```python
from build123d import *
from build123d.topology import SkipClean

# Parameters (mm, degrees)
SKETCH1_W           = 10
SKETCH1_H           = 16
BOSS_EXTRUDE1_DEPTH = 8
FILLET1_R           = 4
SKETCH2_R           = 1.5
CUT_EXTRUDE1_DEPTH  = 16
SKETCH3_W           = 51
SKETCH3_H           = 16
BOSS_EXTRUDE2_DEPTH = 8
SKETCH4_W           = 36
SKETCH4_H           = 16
BOSS_EXTRUDE3_DEPTH = 4.5
SKETCH6_R           = 10.5
CUT_EXTRUDE6_DEPTH  = 16
SKETCH11_W          = 3
SKETCH11_H          = 16
BOSS_EXTRUDE4_DEPTH = 4.5
FILLET3_R           = 4
BOSS_EXTRUDE5_DEPTH = 1
SKETCH14_R          = 1.75
CUT_EXTRUDE7_DEPTH  = 1
BOSS_EXTRUDE6_DEPTH = 5
FILLET4_R           = 6.5
FILLET5_R           = 0.5
FILLET6_R           = 4
FILLET7_R           = 0.5
SKETCH17_W          = 51
SKETCH17_H          = 12.2
CUT_EXTRUDE9_DEPTH  = 6
SKETCH18_R          = 0.5
CUT_EXTRUDE10_DEPTH = 8


# Some blends are built 0.0001 mm under size
with BuildPart() as part:
    # Sketch1 → Boss-Extrude1 (new body)
    with BuildSketch(Plane(origin=(0, 0, 0), x_dir=(1, 0, 0), z_dir=(0, 1, 0))):
        Rectangle(SKETCH1_W, SKETCH1_H)
    extrude(amount=BOSS_EXTRUDE1_DEPTH)

    # Fillet1
    fillet1_edges = [part.edges().sort_by_distance(p)[0] for p in [
        (5, 0, 0),
        (5, 8, 0),
    ]]
    fillet(fillet1_edges, radius=FILLET1_R - 0.0001)  # a hair under: the kernel refuses the full size

    # Sketch2 → Cut-Extrude1 (cut)
    with BuildSketch(Plane.XY.offset(8)):
        with Locations((1, 4)):
            Circle(SKETCH2_R)
    extrude(amount=-CUT_EXTRUDE1_DEPTH, mode=Mode.SUBTRACT)

    # Sketch3 → Boss-Extrude2 (add)
    with BuildSketch(Plane(origin=(0, 0, 0), x_dir=(1, 0, 0), z_dir=(0, 1, 0))):
        with Locations((-30.5, 0)):
            Rectangle(SKETCH3_W, SKETCH3_H)
    extrude(amount=BOSS_EXTRUDE2_DEPTH)

    # Sketch4 → Boss-Extrude3 (add)
    with BuildSketch(Plane(origin=(0, 0, 0), x_dir=(1, 0, 0), z_dir=(0, 1, 0))):
        with Locations((-74, 0)):
            Rectangle(SKETCH4_W, SKETCH4_H)
    extrude(amount=BOSS_EXTRUDE3_DEPTH)

    # Sketch6 → Cut-Extrude6 (cut)
    with BuildSketch(Plane(origin=(0, 4.5, 0), x_dir=(1, 0, 0), z_dir=(0, 1, 0))):
        with Locations((-81.5, 0)):
            Circle(SKETCH6_R)
    extrude(amount=-CUT_EXTRUDE6_DEPTH, mode=Mode.SUBTRACT)


with BuildPart() as cut_extrude6_piece_1:
    # of the separate pieces the step leaves, piece 1, a body of its own (cut_extrude6_pieces)
    add(part.part.solids().sort_by_distance((5, 3.9999, -8))[0])



with BuildPart() as cut_extrude6_piece_2:
    # of the separate pieces the step leaves, piece 2, a body of its own (cut_extrude6_pieces)
    add(part.part.solids().sort_by_distance((-88.300735254, 4.5, 8))[0])



with BuildPart() as cut_extrude6_piece_3:
    # of the separate pieces the step leaves, piece 3, a body of its own (cut_extrude6_pieces)
    add(part.part.solids().sort_by_distance((-88.300735254, 0, -8))[0])


with BuildPart() as cut_extrude6_piece_2_1:
    add(cut_extrude6_piece_2.part)

    add(cut_extrude6_piece_3.part)  # Boss-Extrude4 merges Cut-Extrude6 piece 3
    # Sketch11 → Boss-Extrude4 (add)
    with BuildSketch(Plane(origin=(0, 0, 0), x_dir=(1, 0, 0), z_dir=(0, 1, 0))):
        with Locations((-93.5, 0)):
            Rectangle(SKETCH11_W, SKETCH11_H)
    extrude(amount=BOSS_EXTRUDE4_DEPTH)

    # Fillet3
    fillet3_edges = [cut_extrude6_piece_2_1.edges().sort_by_distance(p)[0] for p in [
        (-95, 2.25, 8),
        (-95, 2.25, -8),
    ]]
    fillet(fillet3_edges, radius=FILLET3_R)


with BuildPart() as cut_extrude6_piece_1_1:
    add(cut_extrude6_piece_1.part)

    add(cut_extrude6_piece_2_1.part)  # Boss-Extrude5 merges Cut-Extrude6 piece 2
    # Sketch13 → Boss-Extrude5 (add)
    with BuildSketch(Plane(origin=(0, 4.5, 0), x_dir=(1, 0, 0), z_dir=(0, 1, 0))):
        with BuildLine():
            Line((-88.300735254, 8), (-91, 8))
            ThreePointArc((-91, 8), (-93.828427125, 6.828427125), (-95, 4))
            Line((-95, 4), (-95, -4))
            ThreePointArc((-95, -4), (-93.828427125, -6.828427125), (-91, -8))
            Line((-91, -8), (-88.300735254, -8))
            Line((-88.300735254, -8), (-74.699264746, -8))
            Line((-74.699264746, -8), (-56, -8))
            Line((-56, -8), (-56, 8))
            Line((-56, 8), (-74.699264746, 8))
            Line((-74.699264746, 8), (-88.300735254, 8))
        make_face()
    extrude(amount=BOSS_EXTRUDE5_DEPTH)

    # Sketch14 → Cut-Extrude7 (cut)
    with BuildSketch(Plane(origin=(0, 5.5, 0), x_dir=(1, 0, 0), z_dir=(0, 1, 0))):
        with Locations(Location((-81.5, 0, 0), (0, 0, 270))):
            Circle(SKETCH14_R)
    extrude(amount=-CUT_EXTRUDE7_DEPTH, mode=Mode.SUBTRACT)

    # Sketch15 → Boss-Extrude6 (add)
    with SkipClean():  # the faces are left unmerged after this step: merging them gives an invalid solid
        with BuildSketch(Plane.XZ):
            with BuildLine():
                Line((-91, 8), (-88.300735254, 8))
                ThreePointArc((-88.300735254, 8), (-92, 0), (-88.300735254, -8))
                Line((-88.300735254, -8), (-91, -8))
                ThreePointArc((-91, -8), (-93.828427125, -6.828427125), (-95, -4))
                Line((-95, -4), (-95, 4))
                ThreePointArc((-95, 4), (-93.828427125, 6.828427125), (-91, 8))
            make_face()
            with BuildLine():
                Line((-71.895313644, 8), (-74.699264746, 8))
                ThreePointArc((-74.699264746, 8), (-71, 0), (-74.699264746, -8))
                Line((-74.699264746, -8), (-71.895313644, -8))
                ThreePointArc((-71.895313644, -8), (-69, 0), (-71.895313644, 8))
            make_face()
        extrude(amount=BOSS_EXTRUDE6_DEPTH)

    # Fillet4
    # the kernel refuses this fillet: 6.5 mm, written as the material it takes off along each edge
    with BuildSketch(Plane(origin=(-81.5, -5, 0), x_dir=(-0.06203986114443866, 0, -0.998073672445666), z_dir=(-0.998073672445666, 0, 0.06203986114443866))) as fillet4_piece_1:
        with BuildLine():
            CenterArc((6, -4.69041576), FILLET4_R, 0, 46.18693854)
            Line((10.5, 0), (12.5, 0))
            Line((12.5, 0), (12.5, -4.69041576))
        make_face()
    revolve(axis=Axis((-81.5, -5, 0), (0, -1, 0)), revolution_arc=187.113812842, mode=Mode.SUBTRACT)

    # Fillet5
    fillet5_edges = [cut_extrude6_piece_1_1.edges().sort_by_distance(p)[0] for p in [
        (-71, 4.5, 0),
        (-92, 4.5, 0),
    ]]
    fillet(fillet5_edges, radius=FILLET5_R)

    # Fillet6
    # the kernel refuses this fillet: 4 mm, written as the material it takes off along each edge
    with BuildSketch(Plane(origin=(-91, -5, 8), x_dir=(0, 0, -1), z_dir=(1, 0, 0))) as fillet6_piece_1:
        with BuildLine():
            CenterArc((FILLET6_R, FILLET6_R), FILLET6_R, 180, 90)
            Line((0, FILLET6_R), (0, 0))
            Line((0, 0), (FILLET6_R, 0))
        make_face()
    extrude(amount=12.699264746, mode=Mode.SUBTRACT)
    with BuildSketch(Plane(origin=(-91, -5, 4), x_dir=(-1, 0, 0), z_dir=(0, 0, -1))) as fillet6_piece_2:
        with BuildLine():
            CenterArc((4 - FILLET6_R, FILLET6_R), FILLET6_R, 270, 90)
            Line((4, FILLET6_R), (4, 0))
            Line((4, 0), (4 - FILLET6_R, 0))
        make_face()
    revolve(axis=Axis((-91, -5, 4), (0, 1, 0)), revolution_arc=90, mode=Mode.SUBTRACT)
    with BuildSketch(Plane(origin=(-78.300735254, -5, -8), x_dir=(0, 1, 0), z_dir=(-1, 0, 0))) as fillet6_piece_3:
        with BuildLine():
            CenterArc((FILLET6_R, -FILLET6_R), FILLET6_R, 90, 90)
            Line((0, -FILLET6_R), (0, 0))
            Line((0, 0), (FILLET6_R, 0))
        make_face()
    extrude(amount=12.699264746, mode=Mode.SUBTRACT)
    with BuildSketch(Plane(origin=(-91, -5, -4), x_dir=(0, 0, -1), z_dir=(1, 0, 0))) as fillet6_piece_4:
        with BuildLine():
            CenterArc((4 - FILLET6_R, FILLET6_R), FILLET6_R, 270, 90)
            Line((4, FILLET6_R), (4, 0))
            Line((4, 0), (4 - FILLET6_R, 0))
        make_face()
    revolve(axis=Axis((-91, -5, -4), (0, 1, 0)), revolution_arc=90, mode=Mode.SUBTRACT)
    with BuildSketch(Plane(origin=(-95, -5, -4), x_dir=(1, 0, 0), z_dir=(0, 0, 1))) as fillet6_piece_5:
        with BuildLine():
            CenterArc((FILLET6_R, FILLET6_R), FILLET6_R, 180, 90)
            Line((0, FILLET6_R), (0, 0))
            Line((0, 0), (FILLET6_R, 0))
        make_face()
    extrude(amount=8, mode=Mode.SUBTRACT)

    # Fillet7
    fillet7_edges = [cut_extrude6_piece_1_1.edges().sort_by_distance(p)[0] for p in [
        (-56, 5.5, 0),
    ]]
    fillet(fillet7_edges, radius=FILLET7_R)

    # Sketch17 → Cut-Extrude9 (cut)
    with BuildSketch(Plane.XZ):
        with Locations((-28.5, 0)):
            Rectangle(SKETCH17_W, SKETCH17_H)
    extrude(amount=-CUT_EXTRUDE9_DEPTH, mode=Mode.SUBTRACT)

    # Sketch18 → Cut-Extrude10 (cut)
    with BuildSketch(Plane.XZ):
        with Locations(Location((-55, 4, 0), (0, 0, 270))):
            Circle(SKETCH18_R)
        with Locations(Location((-55, -4, 0), (0, 0, 270))):
            Circle(SKETCH18_R)
    extrude(amount=-CUT_EXTRUDE10_DEPTH, mode=Mode.SUBTRACT)


solid = cut_extrude6_piece_1_1.part
```
Geometry check sheet. Reference: the model listing, model coordinates, mm. A direction names the side the tool comes from. Coordinates: 2 decimals unless noted, no trailing zeros. Order: outer loops, then holes, each group sorted by start corner. A loop starts at its lowest first (then second) coordinate and runs counter-clockwise, first axis right, second up. Notation, with made-up numbers: (12.5, 56.25) - (43.5, 56.25) arc R26 cw to (43.5, 81.25) - close; hole circle Ø6 at (9.25, 43.5). An arc over 180 degrees is marked (long way). Answer in a Markdown table with one row per item. Add a question column.
1. Section check A-A (x = -81.5). Enter the section's corners in (y, z).
2. Section check C-C (x = -26.5). Enter the section's corners in (y, z).
3. Section check B-B (y = 1.5). Enter the section's corners in (x, z), plus the area to 3 significant figures.
4. Draft check along X on faces 4 (the face through (3.859, 6.797, -0.112)), 5 (the face through (-29, 6, 0)), 6 (the face through (-28, 8, 0)). Enter one of: +X half, -X half, draft (parallel to the pull), parting line (faces both ways), or undercut.
5. Material ranges on L1, parallel to Z at x = -55, y = 2.5; L2, parallel to X at y = 5.05, z = 0; L3, parallel to Z at x = -13, y = 4.5, recorded low to high. Write a range as [from, to].
6. Gauge pin test, flat ends, axial feed: pin 1 Ø6 at (x, z) = (-61.5, 1) entering from +Y; pin 2 Ø5.5 at (x, z) = (-81.5, 0) entering from -Y; pin 3 Ø8 at (x, z) = (-27, 2.5) entering from -Y; pin 4 Ø3 at (y, z) = (0, 5) entering from -X. Record the tip position at first contact, or that the pin passes through.
7. Section check D-D (x = -68). Enter the section's corners in (y, z), plus the area to 3 significant figures.
8. Access from +Z, -Z, +X, -X, +Y, -Y to the whole of each face (thin tool, end or side, straight path). Record for faces 1 (the face through (-3, 3, 0)), 2 (the face through (-76, 5.5, 0)), 3 (the face through (-69.001, -0.153, -0.122)).
Data:
| question | item | result |
|---|---|---|
| 1 | outline | (4.5, -8) - (5.5, -8) - (5.5, -1.75) - (4.5, -1.75) - close; (4.5, 1.75) - (5.5, 1.75) - (5.5, 8) - (4.5, 8) - close |
| 2 | outline | (0, -8) - (8, -8) - (8, 8) - (0, 8) - (0, 6.1) - (6, 6.1) - (6, -6.1) - (0, -6.1) - close |
| 3 | outline | (-95, -4) arc R4 ccw to (-91, -8) - (-88.3, -8) arc R10.5 cw to (-88.3, 8) - (-91, 8) arc R4 ccw to (-95, 4) - close; (-74.7, -8) - (4.12, -8) - (4.12, 8) - (-74.7, 8) arc R10.5 cw to start; hole circle Ø1 at (-55, -4); hole circle Ø1 at (-55, 4); hole (-54, -6.1) - (-3, -6.1) - (-3, 6.1) - (-54, 6.1) - close |
| 3 | area | 656 mm² |
| 4 | face 4 | +X half |
| 4 | face 5 | undercut |
| 4 | face 6 | draft |
| 5 | L1 | z = [-8, -4.5], [-3.5, 3.5], [4.5, 8] |
| 5 | L2 | x = [-95, -83.25], [-79.75, -54], [-3, -0.07], [2.07, 4.86] |
| 5 | L3 | z = [-8, -6.1], [6.1, 8] |
| 6 | pin 1 | stops at y = 5.5 |
| 6 | pin 2 | stops at y = 4.5 |
| 6 | pin 3 | stops at y = 0 |
| 6 | pin 4 | stops at x = -95 |
| 7 | outline | (0, -8) - (5.5, -8) - (5.5, 8) - (0, 8) - close |
| 7 | area | 88.0 mm² |
| 8 | face 1 | -Y |
| 8 | face 2 | +Z, -Z, -X, +Y |
| 8 | face 3 | +X, -Y |
